```python
from build123d import *

# Parameters (mm, degrees)
M12_CLEARANCE_HOLE1_D = 13.5
CIRPATTERN1_COUNT     = 4


with BuildPart() as part:
    # Sketch1 → Revolve1 (revolve)
    with BuildSketch(Plane.XY, mode=Mode.PRIVATE) as revolve1_sk:
        Polygon((-32.477216022, 0), (-32.477216022, 32.5), (11.522783978, 32.5), (11.522783978, 71.5), (21.522783978, 71.5), (21.522783978, 31.5), (72.522783978, 31.5), (72.522783978, 25.5), (98.522783978, 25.5), (98.522783978, 0), align=None)
    revolve(revolve1_sk.sketch.rotate(Axis((98.522783978, 0, 0), (-1, 0, 0)), 90), axis=Axis((98.522783978, 0, 0), (-1, 0, 0)))

    # M12 Clearance Hole1 (through all)
    with Locations(Plane(origin=(21.522783978, 50, 0), x_dir=(0, 0, 1), z_dir=(1, 0, 0))):
        with Locations((0, 0)):
            m12_clearance_hole1 = Hole(M12_CLEARANCE_HOLE1_D / 2)

    # CirPattern1: M12 Clearance Hole1 ×4 about axis
    cirpattern1_axis = Axis((0, 0, 0), (1, 0, 0))
    for i in range(1, CIRPATTERN1_COUNT):
        add(m12_clearance_hole1.rotate(cirpattern1_axis, i * 360 / CIRPATTERN1_COUNT), mode=Mode.SUBTRACT)


solid = part.part
```
The listing builds one solid part. Answer for the finished solid, in the listing's coordinates (mm). A direction names the side the tool comes from. Give positions to 0.01 mm unless a question says otherwise; leave off trailing zeros. Order: outer loops, then holes, each group sorted by start corner. A loop starts at its lowest first (then second) coordinate and runs counter-clockwise, first axis right, second up. Notation, with made-up numbers: (84, -19) - (120, -19) arc R18 cw to (120, 12) - close; hole circle Ø10 at (-39, 60.25). An arc over 180 degrees is marked (long way). Use one line per item in the form item = value. Start each with the question number.
(1) A cutting plane is placed at D-D, the plane x = 55.5. Write down the section's boundary in (y, z).
(2) A cutting plane is placed at B-B, the plane z = 50. Write down the section's boundary in (x, y).
(3) Consider line 1 (Y direction, x = 17, z = 0); line 2 (X direction, y = -40, z = -5); line 3 (X direction, y = -29, z = -8). Determine where each line is inside the solid, lowest interval first. Write a range as from..to.
(4) Flat-ended cylindrical pins translate along their axes: pin 1 Ø8 at (y, z) = (0, 50) entering from -X; pin 2 Ø1.5 at (x, z) = (41, -18.5) entering from -Y; pin 3 Ø4 at (x, z) = (67.5, -4) entering from +Y; pin 4 Ø2 at (y, z) = (-24.5, 39.5) entering from +X. Find the tip coordinate at first contact, or state that the pin passes through.
(5) For faces 4 (the cylindrical face through (85.705, 15.516, 20.236)), 5 (the cylindrical face through (16.59, -48.32, 52.7)), 6 (the flat face through (11.523, 31, 15)), determine the directions among +Z, -Z, +X, -X, +Y, -Y from which every point of the face is accessible in a straight line to the end or side of a thin tool.
(6) The mould has two halves that part along Y. Classify faces 1 (the flat face through (72.523, 0, -26)), 2 (the cylindrical face through (-10.17, -9.76, -31)), 3 (the cylindrical face through (16.45, -55.99, 3.11)): released by +Y, released by -Y, zero draft, split by the parting line, or undercut.
(7) A cutting plane is placed at A-A, the plane x = 14. Write down the section's boundary in (y, z).
Ans:
q1.outline = circle Ø63 at (0, 0)
q2.outline = (11.52, -51.11) - (21.52, -51.11) - (21.52, -6.75) - (11.52, -6.75) - close; (11.52, 6.75) - (21.52, 6.75) - (21.52, 51.11) - (11.52, 51.11) - close
q3.line_1 = -71.5..-56.75, -43.25..43.25, 56.75..71.5
q3.line_2 = 11.52..21.52
q3.line_3 = -32.48..72.52
q4.pin_1 = through
q4.pin_2 = -26.02
q4.pin_3 = 31.44
q4.pin_4 = 21.52
q5.face_4 = +X
q5.face_5 = +X, -X
q5.face_6 = -X
q6.face_1 = zero draft
q6.face_2 = split by the parting line
q6.face_3 = undercut
q7.outline = circle Ø143 at (0, 0); hole circle Ø13.5 at (-50, 0); hole circle Ø13.5 at (0, -50); hole circle Ø13.5 at (0, 50); hole circle Ø13.5 at (50, 0)
